Print and shaded views of the part. All mm, measured from the part's lowest x, y and z. Give positions to 0.01 mm unless a question says otherwise; leave off trailing zeros. Write each loop counter-clockwise with the first axis right and the second up, starting at its lowest first coordinate (ties: lowest second). Pieces come first, ordered by that corner, then holes. Notation, with made-up numbers: M -34,22.5 L -18,22.5 A24 cw -18,46.5 Z; hole C 88,24 d11. An arc over 180 degrees is marked long. One line per question, with ' | ' between items. Start each with the question number.
1. Cut at A-A, the plane x = 10. Write the cut outline in (y, z), then the cut area to 3 significant figures.
2. Flat gauge pin, fed straight in: pin 1 (1 mm diameter, centred on y = 1, z = 40.5, fed in from +X). Where does the tip first touch, or does it go through?
3. Wall check: L1, parallel to Z at x = 10, y = 2.5; L2, parallel to X at y = 1.95, z = 10; L3, parallel to Z at x = 10.5, y = 0.75. Give the ranges that are in metal, low to high.
4. Cut at C-C, the plane y = 1.35. Write the cut outline in (x, z).
5. Cut at D-D, the plane x = 26. Write the cut outline in (y, z).
6. Cut at B-B, the plane z = 10. Write the cut outline in (x, y), then the cut area to 3 significant figures.
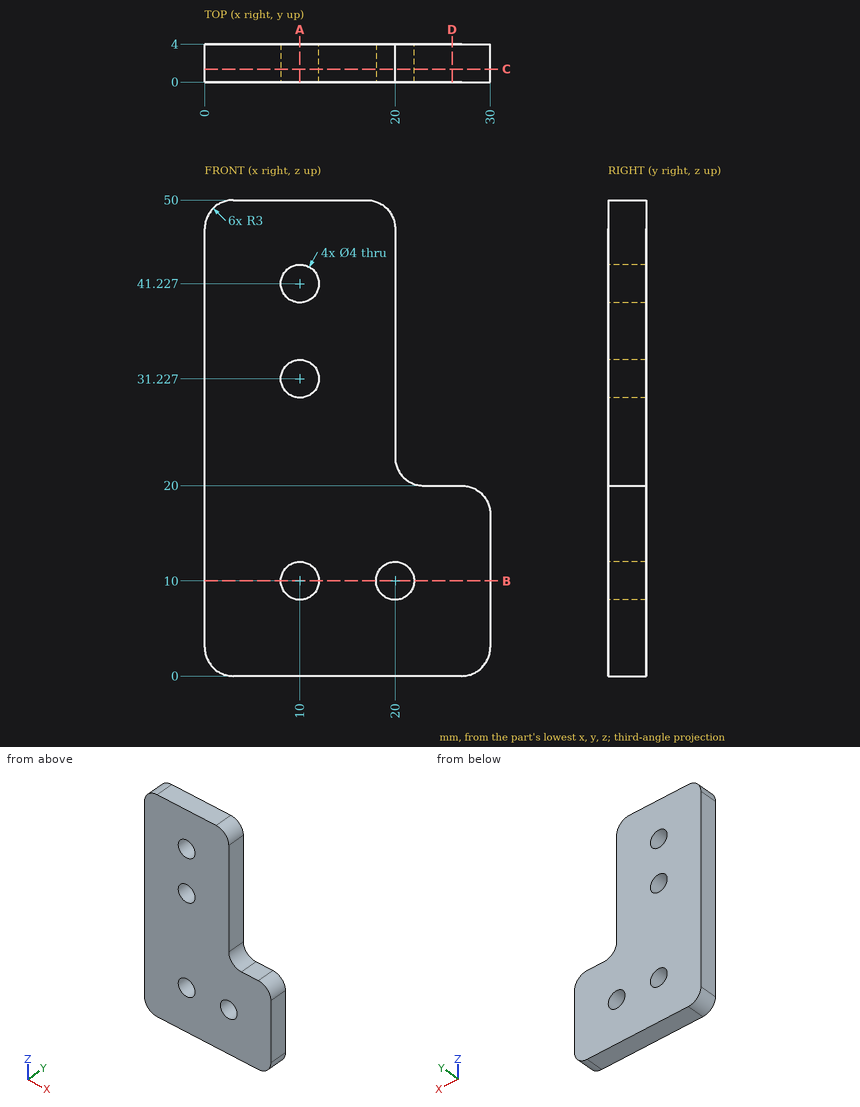
Here are the results:
1) outline: M 0,0 L 4,0 L 4,8 L 0,8 Z; M 0,12 L 4,12 L 4,29.23 L 0,29.23 Z; M 0,33.23 L 4,33.23 L 4,39.23 L 0,39.23 Z; M 0,43.23 L 4,43.23 L 4,50 L 0,50 Z | area: 152 mm^2
2) pin 1: x = 20
3) L1: 0 to 8, 12 to 29.23, 33.23 to 39.23, 43.23 to 50 | L2: 0 to 8, 12 to 18, 22 to 30 | L3: 0 to 8.06, 11.94 to 29.29, 33.16 to 39.29, 43.16 to 50
4) outline: M 0,3 A3 ccw 3,0 L 27,0 A3 ccw 30,3 L 30,17 A3 ccw 27,20 L 23,20 A3 cw 20,23 L 20,47 A3 ccw 17,50 L 3,50 A3 ccw 0,47 Z; hole C 10,10 d4; hole C 10,31.23 d4; hole C 10,41.23 d4; hole C 20,10 d4
5) outline: M 0,0 L 4,0 L 4,20 L 0,20 Z
6) outline: M 0,0 L 8,0 L 8,4 L 0,4 Z; M 12,0 L 18,0 L 18,4 L 12,4 Z; M 22,0 L 30,0 L 30,4 L 22,4 Z | area: 88.0 mm^2
